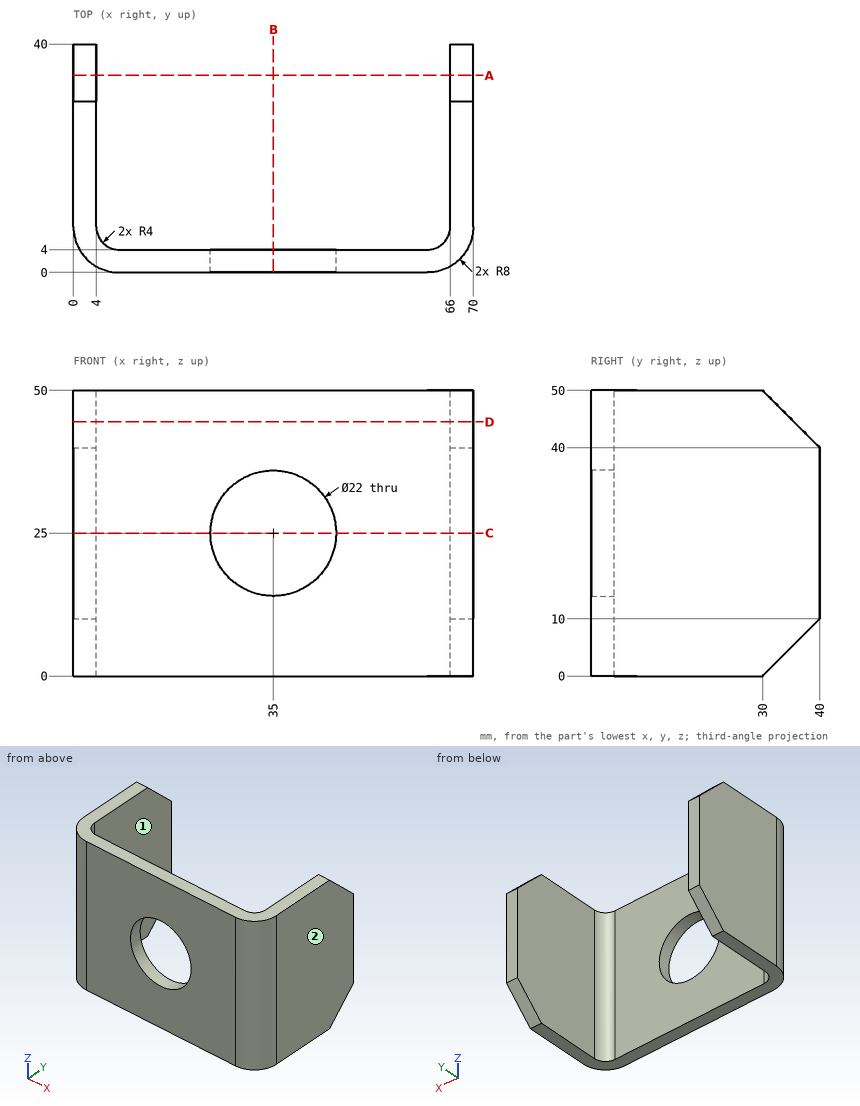
Job drawing, mm, ordinate dimensions from the low corner. One solid piece. A direction names the side the tool comes from. Round coordinates to 2 decimals unless told otherwise and drop trailing zeros. Loops run counter-clockwise (first coordinate to the right, second up) from the corner with the lowest first, then second, coordinate; pieces in that order, holes last.
(1) Cut at B-B (x = 35). Give the cut face in (y, z), plus the area to 3 significant figures.
(2) Wall check: line 1 along X through (y, z) = (33.5, 16); line 2 along Y through (x, z) = (46, 19); line 3 along X through (y, z) = (2.05, 25). Give the ranges that are in metal, low to high.
(3) Which spindle directions (+Z, -Z, +X, -X, +Y, -Y) get a long thin tool onto all of the face, cutting with end or side? Do the marked faces 1 and 2. Say none if no direction does.
(4) Cut at C-C (z = 25). Give the cut face in (x, y).
(5) Drop flat-ended pins along their axis: pin 1 (8 mm diameter, centred on x = 55, y = 9, fed in from +Z); pin 2 (4 mm diameter, centred on y = 9, z = 16, fed in from -X). Give the stop position or say it passes through.
(6) Cut at A-A (y = 34.5). Give the cut face in (x, z).
(7) Cut at D-D (z = 44.5). Give the cut face in (x, y).
Findings below:
1. outline: (0, 0) - (4, 0) - (4, 14) - (0, 14) - close; (0, 36) - (4, 36) - (4, 50) - (0, 50) - close
1. area: 112 mm2
2. line 1: x = 0 to 4, 66 to 70
2. line 2: y = 0 to 4
2. line 3: x = 2.65 to 24, 46 to 67.35
3. face 1: +Z, -Z, +Y
3. face 2: +Z, -Z, +X, +Y, -Y
4. outline: (0, 8) arc R8 ccw to (8, 0) - (24, 0) - (24, 4) - (8, 4) arc R4 cw to (4, 8) - (4, 40) - (0, 40) - close; (46, 0) - (62, 0) arc R8 ccw to (70, 8) - (70, 40) - (66, 40) - (66, 8) arc R4 cw to (62, 4) - (46, 4) - close
5. pin 1: passes through
5. pin 2: stops at x = 0
6. outline: (0, 4.5) - (4, 4.5) - (4, 45.5) - (0, 45.5) - close; (66, 4.5) - (70, 4.5) - (70, 45.5) - (66, 45.5) - close
7. outline: (0, 8) arc R8 ccw to (8, 0) - (62, 0) arc R8 ccw to (70, 8) - (70, 35.5) - (66, 35.5) - (66, 8) arc R4 cw to (62, 4) - (8, 4) arc R4 cw to (4, 8) - (4, 35.5) - (0, 35.5) - close
